Geometry check sheet. Reference: the model listing, model coordinates, mm. Round coordinates to 2 decimals unless told otherwise and drop trailing zeros. Loops run counter-clockwise (first coordinate to the right, second up) from the corner with the lowest first, then second, coordinate; pieces in that order, holes last. Notation, with made-up numbers: (34, 80.25) - (93, 80.25) arc R22 ccw to (93, 110.25) - close; hole circle Ø11 at (54.5, 84.25). An arc over 180 degrees is marked (long way). Answer in a Markdown table with one row per item. Add a question column.
```python
from build123d import *

# Parameters (mm, degrees)
SKETCH1_W                                        = 177.8
SKETCH1_H                                        = 50.8
BOSS_EXTRUDE1_DEPTH                              = 3.175
CSK_FOR_1_4_FLAT_HEAD_MACHINE_SCREW1_D           = 6.7564
CSK_FOR_1_4_FLAT_HEAD_MACHINE_SCREW1_DEPTH       = 19.05
CSK_FOR_1_4_FLAT_HEAD_MACHINE_SCREW1_CSINK_D     = 12.8778
CSK_FOR_1_4_FLAT_HEAD_MACHINE_SCREW1_CSINK_ANGLE = 82
CSK_FOR_1_4_FLAT_HEAD_MACHINE_SCREW1_TIP         = 2.029827343


with BuildPart() as part:
    # Sketch1 → Boss-Extrude1 (new, symmetric)
    with BuildSketch(Plane(origin=(0, 0, 0), x_dir=(1, 0, 0), z_dir=(0, 1, 0))):
        Rectangle(SKETCH1_W, SKETCH1_H)
    extrude(amount=BOSS_EXTRUDE1_DEPTH, both=True)

    # CSK for 1/4 Flat Head Machine Screw1
    with Locations(Plane(origin=(0, 3.175, 0), x_dir=(1, 0, 0), z_dir=(0, 1, 0))):
        with Locations((79.375, 0), (-44.45, 9.525), (-44.45, -9.525)):
            CounterSinkHole(CSK_FOR_1_4_FLAT_HEAD_MACHINE_SCREW1_D / 2, CSK_FOR_1_4_FLAT_HEAD_MACHINE_SCREW1_CSINK_D / 2, depth=CSK_FOR_1_4_FLAT_HEAD_MACHINE_SCREW1_DEPTH, counter_sink_angle=CSK_FOR_1_4_FLAT_HEAD_MACHINE_SCREW1_CSINK_ANGLE)
            with Locations((0, 0, -(CSK_FOR_1_4_FLAT_HEAD_MACHINE_SCREW1_DEPTH + CSK_FOR_1_4_FLAT_HEAD_MACHINE_SCREW1_TIP / 2))):  # 118° drill point
                Cone(0, CSK_FOR_1_4_FLAT_HEAD_MACHINE_SCREW1_D / 2, CSK_FOR_1_4_FLAT_HEAD_MACHINE_SCREW1_TIP, mode=Mode.SUBTRACT)


solid = part.part
```
Q1. Release check for a two-part mould opening along X. For faces 1 (the conical face through (-47.814, -0.175, -10.584)), 2 (the flat face through (-1, 3.175, 0)), 3 (the flat face through (88.9, 0, 0)) record: +X half, -X half, draft (parallel to the pull), parting line (faces both ways), or undercut.
Q2. Cross-section at A-A, the plane x = -44.45. Enter the section's corners in (y, z) (3 decimals), plus the area to 3 significant figures.
Q3. Cross-section at B-B, the plane z = 0. Enter the section's corners in (x, y) (3 decimals).
Q4. Scan lines: line 1 (Z direction, x = -44.45, y = -2.35); line 2 (X direction, y = -1.5, z = -1.5); line 3 (X direction, y = 3, z = -10). Record each from-to range of solid material in increasing order. Write a range as from..to.
Q5. Cross-section at C-C, the plane y = 1.5. Enter the section's corners in (x, z) (3 decimals), plus the area to 3 significant figures.
Check sheet entries:
| question | item | result |
|---|---|---|
| 1 | face 1 | undercut |
| 1 | face 2 | draft |
| 1 | face 3 | +X half |
| 2 | outline | (-3.175, -25.4) - (3.175, -25.4) - (3.175, -15.964) - (-0.346, -12.903) - (-3.175, -12.903) - close; (-3.175, -6.147) - (-0.346, -6.147) - (3.175, -3.086) - (3.175, 3.086) - (-0.346, 6.147) - (-3.175, 6.147) - close; (-3.175, 12.903) - (-0.346, 12.903) - (3.175, 15.964) - (3.175, 25.4) - (-3.175, 25.4) - close |
| 2 | area | 215 mm² |
| 3 | outline | (-88.9, -3.175) - (75.997, -3.175) - (75.997, -0.346) - (72.936, 3.175) - (-88.9, 3.175) - close; (82.753, -3.175) - (88.9, -3.175) - (88.9, 3.175) - (85.814, 3.175) - (82.753, -0.346) - close |
| 4 | line 1 | -25.4..-12.9, -6.15..6.15, 12.9..25.4 |
| 4 | line 2 | -88.9..76.35, 82.4..88.9 |
| 4 | line 3 | -88.9..-50.72, -38.18..88.9 |
| 5 | outline | (-88.9, -25.4) - (88.9, -25.4) - (88.9, 25.4) - (-88.9, 25.4) - close; hole circle Ø9.966 at (-44.45, -9.525); hole circle Ø9.966 at (-44.45, 9.525); hole circle Ø9.966 at (79.375, 0) |
| 5 | area | 8,800 mm² |
